Autodesk Fusion 360 part; units mm, degrees
sketch "Sketch1" plane through (0, 0, 0) normal (0, 0, 1) x (1, 0, 0)
  circle A0 centre (0, 0) radius 101.5
  circle A1 centre (0, 0) radius 16
  circle A2 centre (0, 0) radius 32
  dimension "d1" = 203
  dimension "d2" = 32
  dimension "d3" = 64
extrude "Extrude1" add sketch "Sketch1" along normal blind 51 contours A2
extrude "Extrude2" add sketch "Sketch1" against normal blind 19 contours A0 | A1 | A2
sketch "Sketch2" plane through (0, 0, 0) normal (0, 0, 1) x (1, 0, 0)
  circle A0 centre (0, 0) radius 86
  circle A1 centre (0, 0) radius 32
  circle A2 centre (0, 0) radius 101.5
  circle A3 centre (0, 0) radius 32
  circle A4 centre (-85.9999, 0.1299) radius 8
  dimension "d8" = 172
  dimension "d9" = 64
  dimension "d10" = 64
  dimension "d11" = 203
  dimension "d12" = 64
  dimension "d13" = 16
extrude "Extrude3" cut sketch "Sketch2" against normal blind 30 contours A0 A4 | A0 A4 picked at (-83.3057, 0.1299) picked at (-88.639, 0.1339)
pattern_circular "C-Pattern1" count 6 over 360 about axis through (0, 0, 1.75) along (0, 0, 1) of "Extrude3"
ref_plane "WorkPlane2" through (-117.5, 0, 4.8107) normal (-1, 0, 0) x (0, 1, 0)
ref_plane "WorkPlane3" through (0, 0, 4.8107) normal (-1, 0, 0) x (0, 1, 0)
sketch "Sketch7" plane through (0, 0, 0) normal (0, 0, 1) x (1, 0, 0)
  line L0 (0, 0) -> (0, -117.5)
  circle A0 centre (0, -117.5) radius 6.5
  dimension "d26" = 117.5
  dimension "d27" = 13
extrude "Extrude7" cut sketch "Sketch7" along normal mid plane 16
sketch "Sketch10" plane through (0, 0, 0) normal (1, 0, 0) x (0, 1, 0)
  line L0 (0, 0) -> (-117.5, 0)
  circle A0 centre (-117.5, 0) radius 6.5
  circle A1 centre (-117.5, 0) radius 19
  circle A2 centre (-117.5, 0) radius 6.5
  dimension "d28" = 117.5
  dimension "d29" = 13
  dimension "d30" = 38
sketch "Sketch12" plane through (0, 0, 0) normal (1, 0, 0) x (0, 1, 0)
  line L0 (0, 0) -> (0, 51)
  line L1 (-123.9402, 17.8752) -> (-124.2542, 17.7621)
  circle A0 centre (-117.5, 0) radius 19
  line L2 (-32, 0) -> (-117.5, 0)
  line L3 (-117.5, 0) -> (-117.5, -10)
  line L4 (-117.5, -10) -> (-133.6555, -10)
  line L5 (-32, 51) -> (-123.9402, 17.8752)
  arc A1 (-98.5, 0) -> (-123.9402, 17.8752) centre (-117.5, 0) ccw
  arc A2 (-123.9402, 17.8752) -> (-133.6555, -10) centre (-117.5, 0) ccw
  line L6 (-32, 51) -> (-25, 51)
  line L7 (-25, 51) -> (-25, 0)
  line L8 (-25, 0) -> (-50, 0)
  line L9 (-25, 0) -> (-25, -19)
  line L10 (-25, -19) -> (-117.5, -19)
  dimension "d31" = 51
  dimension "d33" = 51
  dimension "d40" = 19
extrude "Extrude9" add sketch "Sketch12" along normal mid plane 16
extrude "Extrude8" cut sketch "Sketch10" along normal mid plane 16 contours A0 A2
pattern_circular "C-Pattern2" count 3 over 360 about axis through (0, 0, 0) along (0, 0, 1) of "Extrude8", "Extrude9"
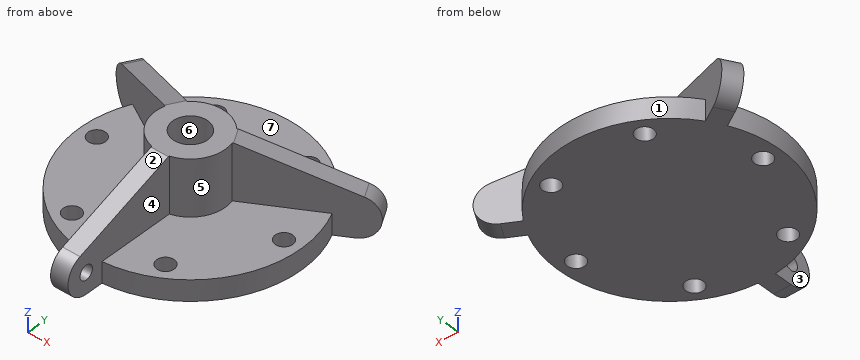
Check sheet for the modelled part. Datum: model origin and axes. Units: mm. Face numbers are marked on the shaded views. A direction names the side the tool comes from. Coordinates: 2 decimals unless noted, no trailing zeros. Order: outer loops, then holes, each group sorted by start corner. A loop starts at its lowest first (then second) coordinate and runs counter-clockwise, first axis right, second up. Notation, with made-up numbers: M 55.25,53 L 80.25,53 A17 cw 80.25,81 Z; hole C 74,-27 d2. An arc over 180 degrees is marked long. Write each question's results on one line, items separated by ' | '. Start each with the question number.
1. Cross-section at B-B on z = 25.5. Record the cut outline in (x, y).
2. Access from +Z, -Z, +X, -X, +Y, -Y to the whole of each face (thin tool, end or side, straight path). Record for the marked faces 4, 5, 6 and 7.
3. Cross-section at A-A on x = 0. Record the cut outline in (y, z), and give its area (3 significant figures).
4. Go/stop test with flat-tipped pins: P1, Ø8, axis at x = -17.5, z = 29, coming from the -Y side; P2, Ø1, axis at y = 10.5, z = 30, coming from the -X side; P3, Ø21, axis at x = -86, y = 0.13, coming from the +Z side; P4, Ø18.5, axis at x = 86, y = -0.13, coming from the -Z side. Record where each tip stops, or that it passes through.
5. Cross-section at D-D on y = 39. Record the cut outline in (x, z).
6. Mould release check, pull along X, two halves, no side actions. Record for the marked faces 1, 2 and 3: +X half, -X half, draft (parallel to the pull), parting line (faces both ways), or undercut.
7. Material ranges on probe 1 along X at (y, z) = (-6, -1); probe 2 along X at (y, z) = (5.5, -9); probe 3 along Z at (x, y) = (26, -60), recorded low to high.
8. Cross-section at C-C on x = 48. Record the cut outline in (y, z).
Checks:
1) outline: M -93.01,44.46 L -30.83,8.56 A32 ccw -8,-30.98 L -8,-102.78 L 8,-102.78 L 8,-30.98 A32 ccw 30.83,8.56 L 93.01,44.46 L 85.01,58.32 L 22.83,22.42 A32 ccw -22.83,22.42 L -85.01,58.32 Z; hole C 0,0 d32
2) face 4: +Z, +X, -Y | face 5: +Z, +X | face 6: +Z | face 7: +Z, +Y
3) outline: M -123.94,17.88 A19 ccw -117.5,-19 L 101.5,-19 L 101.5,0 L 32,0 L 32,51 L 16,51 L 16,0 L -16,0 L -16,51 L -32,51 Z; hole C -117.5,0 d13 | area: 9,270 mm²
4) P1: stops at y = -29.01 | P2: stops at x = -35.05 | P3: stops at z = 0 | P4: stops at z = -19
5) outline: M -93.71,-19 L 93.71,-19 L 93.71,0 L 83.55,0 L 83.55,29.43 L 51.55,39.42 L 51.55,0 L -51.55,0 L -51.55,39.42 L -83.55,29.43 L -83.55,0 L -93.71,0 Z
6) face 1: undercut | face 2: draft | face 3: -X half
7) probe 1: x = -101.32 to -91.14, -80.86 to 80.56, 91.44 to 101.32 | probe 2: x = -101.35 to -91.93, -80.07 to 80.32, 91.68 to 101.35 | probe 3: z = -19 to 0
8) outline: M -89.43,-19 L -80.7,-19 L -80.7,0 L -89.43,0 Z; M -68.39,-19 L 68.08,-19 L 68.08,0 L 36.95,0 L 36.95,40.9 L 18.48,44.22 L 18.48,0 L -68.39,0 Z; M 80.75,-19 L 89.43,-19 L 89.43,0 L 80.75,0 Z
